Design review of the part shown in the three views and the two pictorial views. Dimensions are in mm from the part's minimum x, y and z. A direction names the side the tool comes from. Round coordinates to 2 decimals unless told otherwise and drop trailing zeros. Loops run counter-clockwise (first coordinate to the right, second up) from the corner with the lowest first, then second, coordinate; pieces in that order, holes last. Notation, with made-up numbers: (-18.5, -20.5) -> (-8.5, -20.5) arc R11 cw to (-8.5, -11.5) -> close; hole circle Ø9 at (7.5, 39). An arc over 180 degrees is marked (long way). Use a Markdown table: item, result. Add a question column.
1) Wall thickness on probe 1 along Y at (x, z) = (15.81, 24.35) (3 decimals); probe 2 along Z at (x, y) = (7, 4); probe 3 along X at (y, z) = (30, 24.25): over which ranges is each line inside the solid? List them lowest first.
2) Mouldability with a two-part tool opening along X and no side actions: class the marked faces 6, 7 and 8 as released by +X, released by -X, zero draft, split by the parting line, or undercut.
3) Consider section D-D on y = 13.5. Give the boundary of the cut face in (x, z).
4) Insertion check: pin 1 (12 mm diameter, centred on y = 33.5, z = 12.5, fed in from +X); pin 2 (5 mm diameter, centred on x = 23, z = 18.5, fed in from +Y); pin 3 (3.5 mm diameter, centred on y = 8.5, z = 4.5, fed in from -X); pin 4 (3 mm diameter, centred on x = 18, z = 6.5, fed in from +Y). Each pin has a flat end and moves straight along its axis. Give the tip position at first contact, or say it passes through.
5) Consider section A-A on x = 15.81. Give the boundary of the cut face in (y, z) (3 decimals), plus the area to 3 significant figures.
6) Consider section C-C on x = 5.5. Give the boundary of the cut face in (y, z).
7) For the marked faces 1, 2, 3, 4 and 5, list the 3-axis set-ups (+Z, -Z, +X, -X, +Y, -Y) from which the entire face can be reached by the end or side of a thin tool; tool diameter is ignored.
8) Consider section B-B on y = 37.5. Give the boundary of the cut face in (x, z), plus the area to 3 significant figures.
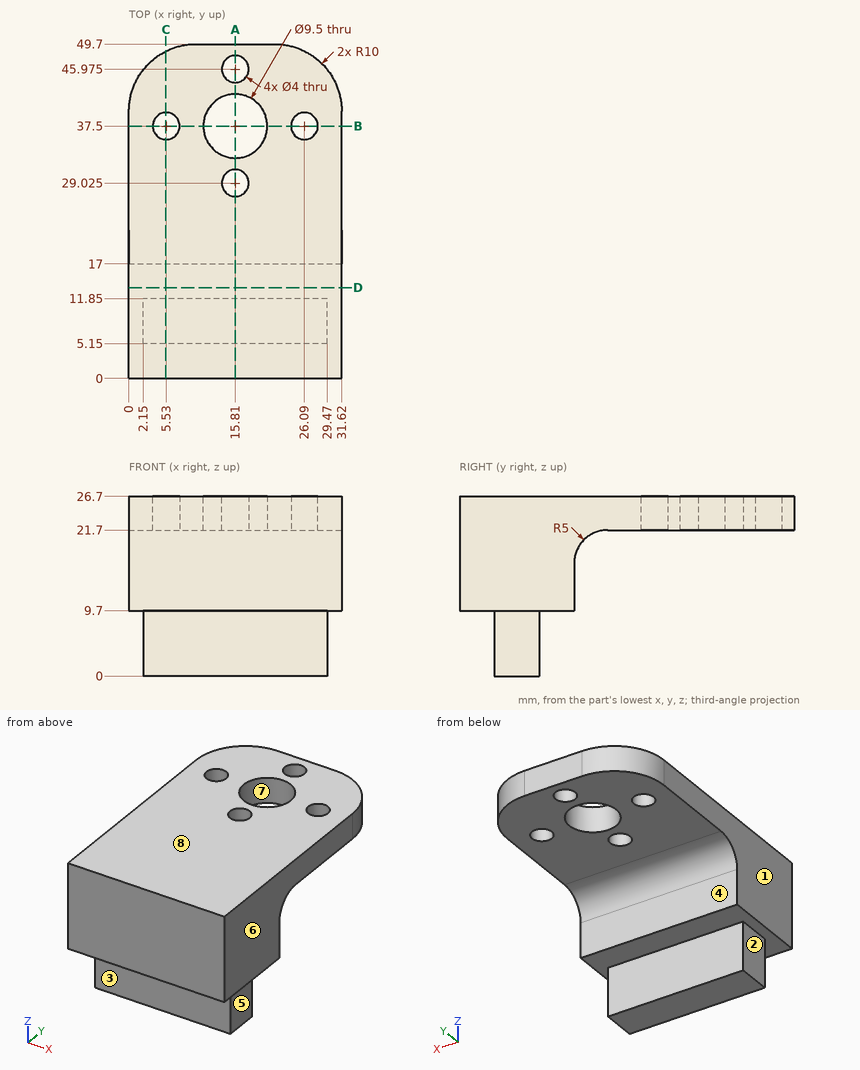
Result set:
| question | item | result |
|---|---|---|
| 1 | probe 1 | 0 to 27.025, 31.025 to 32.75, 42.25 to 43.975, 47.975 to 49.7 |
| 1 | probe 2 | 9.7 to 26.7 |
| 1 | probe 3 | 0 to 14.06, 17.56 to 31.62 |
| 2 | face 6 | released by +X |
| 2 | face 7 | undercut |
| 2 | face 8 | zero draft |
| 3 | outline | (0, 9.7) -> (31.62, 9.7) -> (31.62, 26.7) -> (0, 26.7) -> close |
| 4 | pin 1 | through |
| 4 | pin 2 | y = 19.45 |
| 4 | pin 3 | x = 2.15 |
| 4 | pin 4 | y = 11.85 |
| 5 | outline | (0, 9.7) -> (5.15, 9.7) -> (5.15, 0) -> (11.85, 0) -> (11.85, 9.7) -> (17, 9.7) -> (17, 16.7) arc R5 cw to (22, 21.7) -> (27.025, 21.7) -> (27.025, 26.7) -> (0, 26.7) -> close; (31.025, 21.7) -> (32.75, 21.7) -> (32.75, 26.7) -> (31.025, 26.7) -> close; (42.25, 21.7) -> (43.975, 21.7) -> (43.975, 26.7) -> (42.25, 26.7) -> close; (47.975, 21.7) -> (49.7, 21.7) -> (49.7, 26.7) -> (47.975, 26.7) -> close |
| 5 | area | 435 mm2 |
| 6 | outline | (0, 9.7) -> (5.15, 9.7) -> (5.15, 0) -> (11.85, 0) -> (11.85, 9.7) -> (17, 9.7) -> (17, 16.7) arc R5 cw to (22, 21.7) -> (35.5, 21.7) -> (35.5, 26.7) -> (0, 26.7) -> close; (39.5, 21.7) -> (48.63, 21.7) -> (48.63, 26.7) -> (39.5, 26.7) -> close |
| 7 | face 1 | +Z, -Z, -X, +Y, -Y |
| 7 | face 2 | -Z, -X, +Y, -Y |
| 7 | face 3 | -Z, +X, -X, -Y |
| 7 | face 4 | -Z, +X, -X, +Y |
| 7 | face 5 | -Z, +X, +Y, -Y |
| 8 | outline | (0, 21.7) -> (3.53, 21.7) -> (3.53, 26.7) -> (0, 26.7) -> close; (7.53, 21.7) -> (11.06, 21.7) -> (11.06, 26.7) -> (7.53, 26.7) -> close; (20.56, 21.7) -> (24.09, 21.7) -> (24.09, 26.7) -> (20.56, 26.7) -> close; (28.09, 21.7) -> (31.62, 21.7) -> (31.62, 26.7) -> (28.09, 26.7) -> close |
| 8 | area | 70.6 mm2 |
